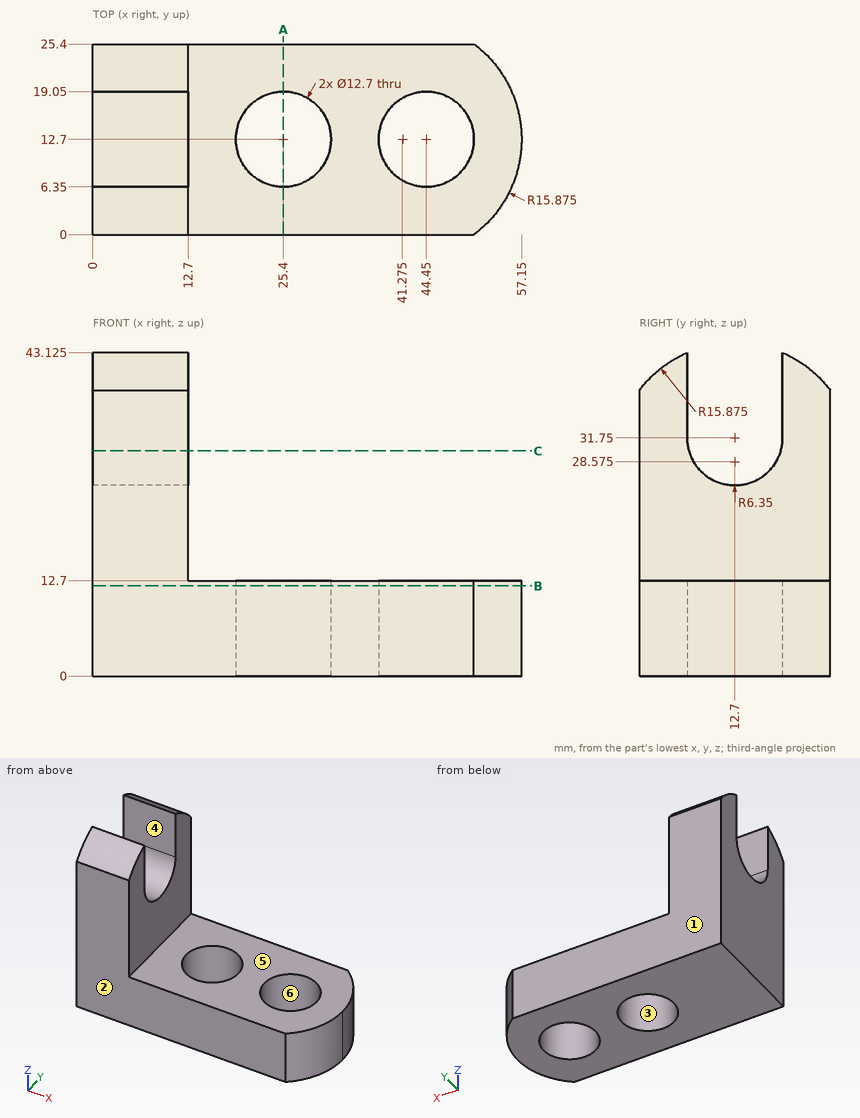
Drawing for the job (mm, zero at the part's lowest x, y, z). A direction names the side the tool comes from. Give positions to 0.01 mm unless a question says otherwise; leave off trailing zeros. Write each loop counter-clockwise with the first axis right and the second up, starting at its lowest first coordinate (ties: lowest second). Pieces come first, ordered by that corner, then holes. Notation, with made-up numbers: M 57,86 L 116,86 A24 cw 116,112 Z; hole C 88.5,-24.5 d3. An arc over 180 degrees is marked long. Return JSON: item names as keys, results as strings. Group by question number.
(1) 3-axis set-ups, long thin cutter, end or side, ignore diameter. For the marked faces 4, 5 and 6: which of +Z, -Z, +X, -X, +Y, -Y reach the whole face in a straight line?
(2) Band-saw the part on C-C (z = 30). Give the cut face in (x, y).
(3) Drill centre lines: L1, parallel to Y at x = 25.4, z = 8.5; L2, parallel to Z at x = 26, y = 1.75; L3, parallel to Y at x = 41.5, z = 9. Where is each one in solid material? Low to high. Write a range as [from, to].
(4) Band-saw the part on A-A (x = 25.4). Give the cut face in (y, z).
(5) Flat gauge pins, fed straight in: pin 1 Ø3 at (x, y) = (27.5, 10.5) entering from +Z; pin 2 Ø3 at (x, y) = (48, 22) entering from +Z; pin 3 Ø1.5 at (y, z) = (19.5, 6) entering from +X; pin 4 Ø5 at (y, z) = (17.5, 31.5) entering from +X. Where does each tip first touch, or does it go through?
(6) Mould opens along Y. For the marked faces 1, 2 and 3 say: pulls with the +Y half, pulls with the -Y half, needs draft (parallel to the pull), parting line crosses it, or undercut.
(7) Band-saw the part on B-B (z = 12). State how many separate pieces and enclosed holes the cut face has, and give its area (3 significant figures).
Entries:
{
 "1": {"face 4": "+Z, +X, -X", "face 5": "+Z, +X, +Y, -Y", "face 6": "+Z, -Z"},
 "2": {"outline": "M 0,0 L 12.7,0 L 12.7,6.6 L 0,6.6 Z; M 0,18.8 L 12.7,18.8 L 12.7,25.4 L 0,25.4 Z"},
 "3": {"L1": "y = [0, 6.35], [19.05, 25.4]", "L2": "z = [0, 12.7]", "L3": "y = [0, 7.08], [18.32, 25.4]"},
 "4": {"outline": "M 0,0 L 6.35,0 L 6.35,12.7 L 0,12.7 Z; M 19.05,0 L 25.4,0 L 25.4,12.7 L 19.05,12.7 Z"},
 "5": {"pin 1": "passes through", "pin 2": "stops at z = 12.7", "pin 3": "stops at x = 55.95", "pin 4": "stops at x = 12.7"},
 "6": {"face 1": "pulls with the +Y half", "face 2": "pulls with the -Y half", "face 3": "undercut"},
 "7": {"separate pieces": "1", "enclosed holes": "2", "area": "1,150 mm^2"}
}
